Geometry: see drawing. Coordinates: mm, zero at the bounding-box minimum. A direction names the side the tool comes from. Round coordinates to 2 decimals unless told otherwise and drop trailing zeros. Loops run counter-clockwise (first coordinate to the right, second up) from the corner with the lowest first, then second, coordinate; pieces in that order, holes last.
(1) Cut plane B-B, the plane y = 8. Output: boundary loops of the cut face in (x, z), and give its area (3 significant figures).
(2) Cut plane C-C, the plane x = 19.5. Output: boundary loops of the cut face in (y, z).
(3) Draft query along X for the marked faces 1, 2, 3 and 4. Return one class per face: released by +X, released by -X, zero draft, split by the parting line, or undercut.
(4) First-contact query: pin 1 Ø2 at (x, y) = (14, 10.5) entering from -Z; pin 2 Ø3 at (x, z) = (5.5, 7) entering from -Y; pin 3 Ø4.5 at (x, y) = (11.5, 2.5) entering from -Z. Flat tips, straight axial feed; report the tip coordinate or a pass-through.
(5) Cut plane A-A, the plane z = 11.5. Output: boundary loops of the cut face in (x, y).
(6) Access query for the marked faces 5, 6 and 7. Directions: +Z, -Z, +X, -X, +Y, -Y. A direction counts if a zero-diameter tool reaches every point of the face in a straight line with its end or side. Return the directions, or none.
(7) Cut plane D-D, the plane y = 3.75. Output: boundary loops of the cut face in (x, z), and give its area (3 significant figures).
(8) Line query: line 1 (X direction, y = 8.3, z = 11.5); line 2 (Y direction, x = 6.25, z = 7.75); line 3 (Y direction, x = 11.5, z = 16.25). Output: solid intervals per line, ascending.
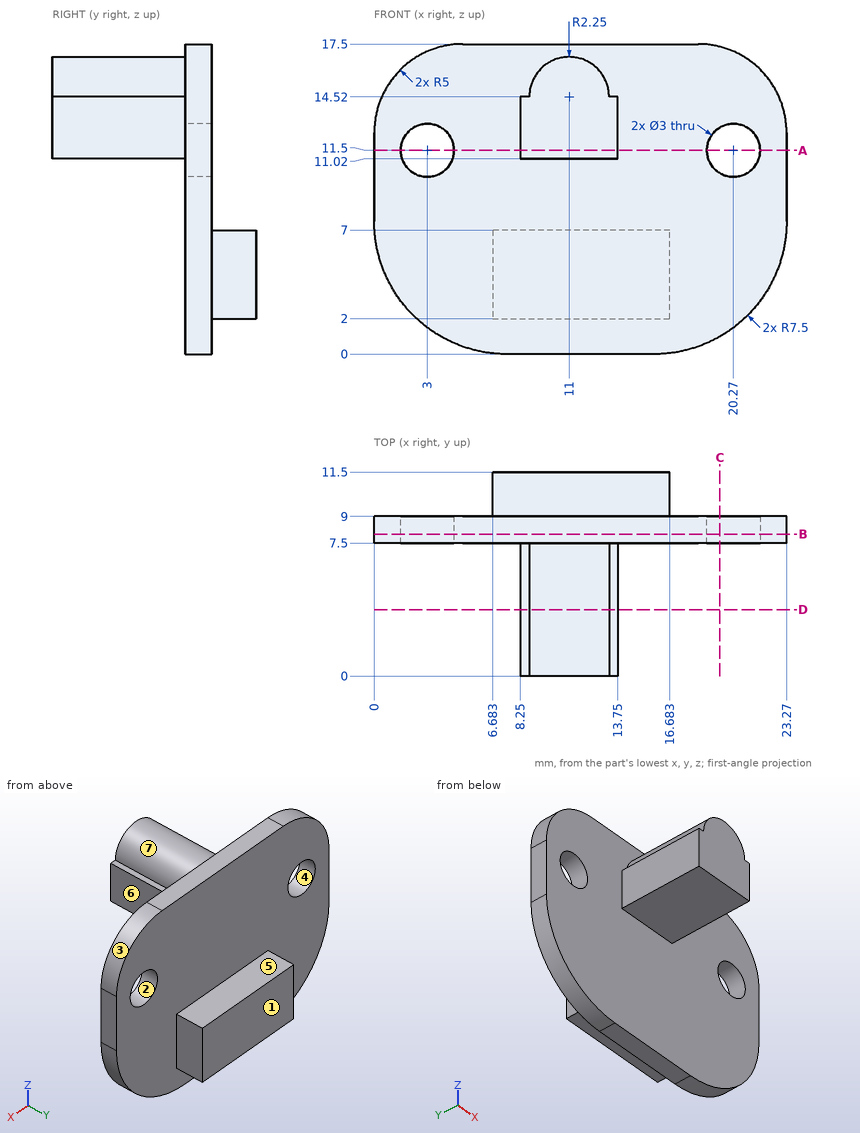
Reported:
1. outline: (0, 7.5) arc R7.5 ccw to (7.5, 0) - (15.77, 0) arc R7.5 ccw to (23.27, 7.5) - (23.27, 12.5) arc R5 ccw to (18.27, 17.5) - (5, 17.5) arc R5 ccw to (0, 12.5) - close; hole circle Ø3 at (3, 11.5); hole circle Ø3 at (20.27, 11.5)
1. area: 358 mm2
2. outline: (7.5, 0.99) - (9, 0.99) - (9, 10.21) - (7.5, 10.21) - close; (7.5, 12.79) - (9, 12.79) - (9, 17.35) - (7.5, 17.35) - close
3. face 1: zero draft
3. face 2: undercut
3. face 3: released by +X
3. face 4: undercut
4. pin 1: stops at z = 2
4. pin 2: stops at y = 7.5
4. pin 3: stops at z = 11.02
5. outline: (0, 7.5) - (1.5, 7.5) - (1.5, 9) - (0, 9) - close; (4.5, 7.5) - (8.25, 7.5) - (8.25, 0) - (13.75, 0) - (13.75, 7.5) - (18.77, 7.5) - (18.77, 9) - (4.5, 9) - close; (21.77, 7.5) - (23.27, 7.5) - (23.27, 9) - (21.77, 9) - close
6. face 5: +Z, +X, -X, +Y
6. face 6: +Z, -Z, +X, -Y
6. face 7: +Z, -Y
7. outline: (8.25, 11.02) - (13.75, 11.02) - (13.75, 14.52) - (13.25, 14.52) arc R2.25 ccw to (8.75, 14.52) - (8.25, 14.52) - close
7. area: 27.2 mm2
8. line 1: x = 0 to 1.5, 4.5 to 18.77, 21.77 to 23.27
8. line 2: y = 7.5 to 9
8. line 3: y = 0 to 9
